```python
from build123d import *

# Parameters (mm, degrees)
SKETCH_R   = 4
SKETCH_R_2 = 2.75
PAD_DEPTH  = 5


with BuildPart() as part:
    # Sketch → Pad (new body, symmetric)
    with BuildSketch(Plane.XY):
        with BuildLine():
            ThreePointArc((18.848305, -4.543015), (21.76, 0), (18.848305, 4.543014))
            Line((5.011933, 10.903235), (18.848305, 4.543014))
            ThreePointArc((5.011933, 10.903235), (0, 12), (-5.011933, 10.903235))
            Line((-18.848305, 4.543014), (-5.011933, 10.903235))
            ThreePointArc((-18.848305, 4.543014), (-21.76, 1.3e-05), (-18.848328, -4.543004))
            Line((-18.848328, -4.543004), (-5.011941, -10.903231))
            ThreePointArc((-5.011941, -10.903231), (-1.2e-05, -12), (5.01192, -10.903241))
            Line((5.01192, -10.903241), (18.848305, -4.543015))
        make_face()
        Circle(SKETCH_R, mode=Mode.SUBTRACT)
        with Locations((-16, 0)):
            Circle(SKETCH_R_2, mode=Mode.SUBTRACT)
        with Locations((16, 0)):
            Circle(SKETCH_R_2, mode=Mode.SUBTRACT)
    extrude(amount=PAD_DEPTH, both=True)


solid = part.part
```
Build history of the part. All positions in model axes, mm. Coordinates: 2 decimals unless noted, no trailing zeros. Order: outer loops, then holes, each group sorted by start corner. A loop starts at its lowest first (then second) coordinate and runs counter-clockwise, first axis right, second up. Notation, with made-up numbers: M 55,47.5 L 101,47.5 A25 cw 101,70.5 Z; hole C 77.5,81.5 d7. An arc over 180 degrees is marked long. One line per question, with ' | ' between items. Start each with the question number.
1. Cut at A-A (x = 0). Write the cut outline in (y, z).
2. Flat gauge pins, fed straight in: P1, Ø4, axis at x = 14, z = -0.5, coming from the +Y side; P2, Ø3.5, axis at x = -16, y = 0, coming from the +Z side; P3, Ø4, axis at y = 5.5, z = -1.5, coming from the +X side. Where does each tip first touch, or does it go through?
3. Cut at D-D (x = 15). Write the cut outline in (y, z), plus the area to 3 significant figures.
4. Cut at C-C (y = -1.5). Write the cut outline in (x, z).
5. Wall check: line 1 along Y through (x, z) = (0, 2.25); line 2 along X through (y, z) = (-2, -3.25); line 3 along Y through (x, z) = (5, 0.5). Give the ranges that are in metal, low to high. Write a range as [from, to].
6. Cut at B-B (z = 2.75). Write the cut outline in (x, y), plus the area to 3 significant figures.
7. Mould opens along X. For faces 1 (the face through (-18.747, 0.121, -0.07)), 2 (the face through (-5, 0, 5)), 3 (the face through (-12.027, -7.679, 0.07)) say: +X half, -X half, draft (parallel to the pull), parting line (faces both ways), or undercut.
The answers:
1) outline: M -12,-5 L -4,-5 L -4,5 L -12,5 Z; M 4,-5 L 12,-5 L 12,5 L 4,5 Z
2) P1: stops at y = 7.69 | P2: passes through | P3: stops at x = 20.33
3) outline: M -6.31,-5 L -2.56,-5 L -2.56,5 L -6.31,5 Z; M 2.56,-5 L 6.31,-5 L 6.31,5 L 2.56,5 Z | area: 75.0 mm2
4) outline: M -21.53,-5 L -18.3,-5 L -18.3,5 L -21.53,5 Z; M -13.7,-5 L -3.71,-5 L -3.71,5 L -13.7,5 Z; M 3.71,-5 L 13.7,-5 L 13.7,5 L 3.71,5 Z; M 18.3,-5 L 21.53,-5 L 21.53,5 L 18.3,5 Z
5) line 1: y = [-12, -4], [4, 12] | line 2: x = [-21.34, -17.89], [-14.11, -3.46], [3.46, 14.11], [17.89, 21.34] | line 3: y = [-10.91, 10.91]
6) outline: M -18.85,-4.54 L -5.01,-10.9 A12 ccw 5.01,-10.9 L 18.85,-4.54 A5 ccw 18.85,4.54 L 5.01,10.9 A12 ccw -5.01,10.9 L -18.85,4.54 A5 ccw Z; hole C -16,0 d5.5; hole C 0,0 d8; hole C 16,0 d5.5 | area: 601 mm2
7) face 1: undercut | face 2: draft | face 3: -X half
